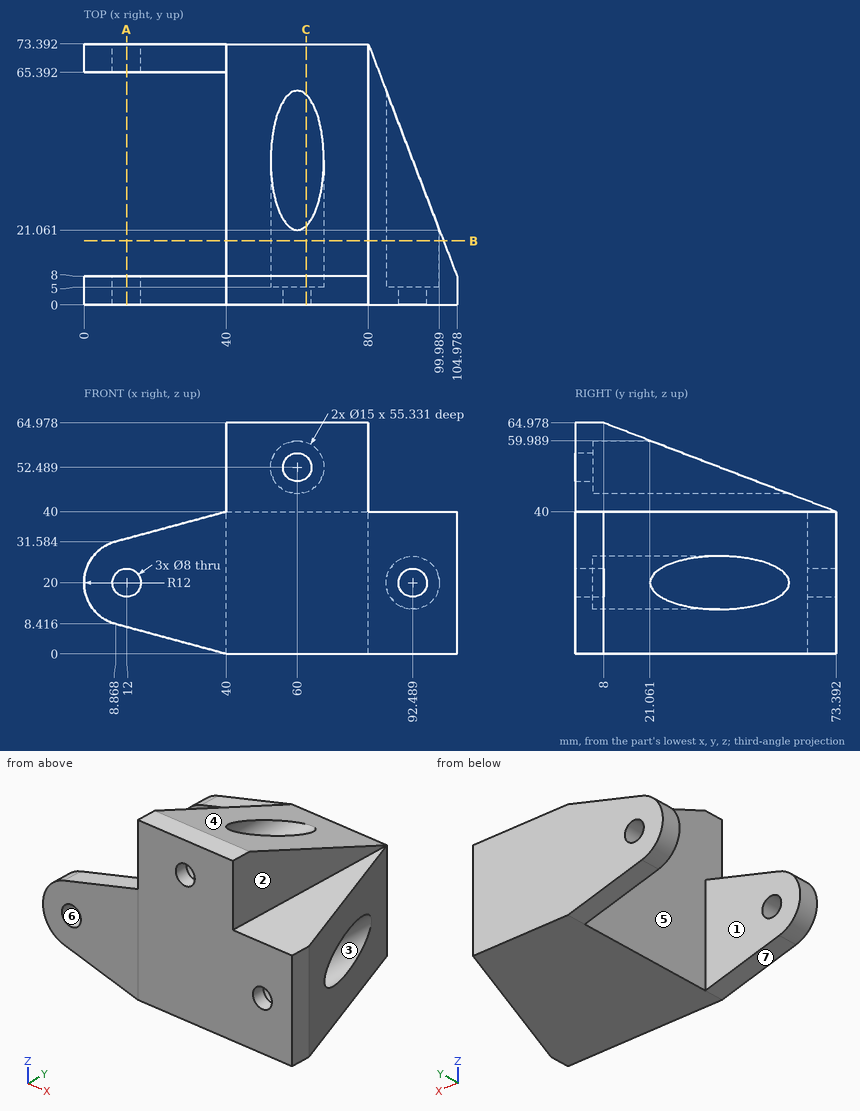
Input: dimensioned drawing with shaded views. Units: mm. Origin: part minimum x, y, z. A direction names the side the tool comes from. Coordinates: 2 decimals unless noted, no trailing zeros. Loops run counter-clockwise (first coordinate to the right, second up) from the corner with the lowest first, then second, coordinate; pieces in that order, holes last. Notation, with made-up numbers: M 20,-21.5 L 41,-21.5 A18 ccw 41,-2.5 Z; hole C 35.25,65 d10. An arc over 180 degrees is marked long. Use a Markdown table: item, result. Add a question column.
Q1. First-contact query: pin 1 (6 mm diameter, centred on x = 58.5, y = 19.5, fed in from +Z); pin 2 (12.5 mm diameter, centred on y = 30, z = 53, fed in from +X); pin 3 (1 mm diameter, centred on y = 14, z = 10.5, fed in from +X); pin 4 (13.5 mm diameter, centred on x = 60, z = 52.49, fed in from -Y). Flat tips, straight axial feed; report the tip coordinate or a pass-through.
Q2. Section query C-C, the plane x = 62.5. Return loops of the section in (y, z) (1 decimal).
Q3. Material intervals for L1, parallel to X at y = 3.4, z = 20; L2, parallel to Y at x = 8, z = 27; L3, parallel to X at y = 7, z = 19.5 (1 decimal), sorted ascending.
Q4. Section query B-B, the plane y = 18. Return loops of the section in (x, z), and give its area (3 significant figures).
Q5. Draft query along Z for the marked faces 4, 5, 6 and 7. Return one class per face: pulls with the +Z half, pulls with the -Z half, needs draft (parallel to the pull), parting line crosses it, or undercut.
Q6. Access query for the marked faces 1, 2 and 3. Directions: +Z, -Z, +X, -X, +Y, -Y. A direction counts if a zero-diameter tool reaches every point of the face in a straight line with its end or side. Return the directions, or none.
Q7. Section query A-A, the plane x = 12. Return loops of the section in (y, z), and give its area (3 significant figures).
Result:
| question | item | result |
|---|---|---|
| 1 | pin 1 | stops at z = 61.73 |
| 1 | pin 2 | stops at x = 80 |
| 1 | pin 3 | stops at x = 102.88 |
| 1 | pin 4 | stops at y = 0 |
| 2 | outline | M 0,0 L 73.4,0 L 73.4,40 L 59.2,45.4 L 5,45.4 L 5,49.4 L 0,49.4 Z; M 0,55.6 L 5,55.6 L 5,59.6 L 22.2,59.6 L 8,65 L 0,65 Z |
| 3 | L1 | x = 0 to 8, 16 to 88.49, 96.49 to 104.98 |
| 3 | L2 | y = 0 to 8, 65.39 to 73.39 |
| 3 | L3 | x = 0 to 8, 16 to 85, 100 to 105 |
| 4 | outline | M 40,0 L 101.16,0 L 101.16,40 L 80,40 L 80,61.16 L 40,61.16 Z; hole C 60,52.49 d15; hole C 92.49,20 d15 |
| 4 | area | 2,940 mm2 |
| 5 | face 4 | pulls with the +Z half |
| 5 | face 5 | needs draft |
| 5 | face 6 | undercut |
| 5 | face 7 | pulls with the -Z half |
| 6 | face 1 | +Z, -Z, -X |
| 6 | face 2 | +Z, +X, +Y, -Y |
| 6 | face 3 | +Y |
| 7 | outline | M 0,7.57 L 8,7.57 L 8,16 L 0,16 Z; M 0,24 L 8,24 L 8,32.43 L 0,32.43 Z; M 65.39,7.57 L 73.39,7.57 L 73.39,16 L 65.39,16 Z; M 65.39,24 L 73.39,24 L 73.39,32.43 L 65.39,32.43 Z |
| 7 | area | 270 mm2 |
